Part model, mm, in its own coordinate system. A direction names the side the tool comes from. Give positions to 0.01 mm unless a question says otherwise; leave off trailing zeros. Loops run counter-clockwise (first coordinate to the right, second up) from the corner with the lowest first, then second, coordinate; pieces in that order, holes last. Notation, with made-up numbers: M 73,-28.75 L 122,-28.75 A12 cw 122,-11.75 Z; hole C -37.75,70.25 d3. An arc over 180 degrees is marked long. Answer in a Markdown table with one row per item.
from build123d import *

# Parameters (mm, degrees)
SKETCH1_R           = 2.5
BOSS_EXTRUDE1_DEPTH = 15
SKETCH3_W           = 4
SKETCH3_H           = 5
CUT_EXTRUDE1_START  = -1
CUT_EXTRUDE1_DEPTH  = 30
CHAMFER1_SIZE       = 0.5


with BuildPart() as part:
    # Sketch1 → Boss-Extrude1 (new body)
    with BuildSketch(Plane(origin=(0, 0, 0), x_dir=(1, 0, 0), z_dir=(0, 1, 0))):
        with Locations(Location((0, 0, 0), (0, 0, 270))):
            Circle(SKETCH1_R)
    extrude(amount=BOSS_EXTRUDE1_DEPTH)

    # Sketch3 → Revolve1 (revolve)
    with BuildSketch(Plane.XY, mode=Mode.PRIVATE) as revolve1_sk:
        with Locations((-2, -2.5)):
            Rectangle(SKETCH3_W, SKETCH3_H)
    revolve(revolve1_sk.sketch.rotate(Axis((0, -5, 0), (0, 1, 0)), 270), axis=Axis((0, -5, 0), (0, 1, 0)))

    # Sketch4 → Cut-Extrude1 (cut)
    with BuildSketch(Plane(origin=(0, 0, 0), x_dir=(1, 0, 0), z_dir=(0, 1, 0)).offset(CUT_EXTRUDE1_START)):
        Polygon((2.886751346, 0), (1.443375673, 2.5), (-1.443375673, 2.5), (-2.886751346, 0), (-1.443375673, -2.5), (1.443375673, -2.5), align=None)
    extrude(amount=-CUT_EXTRUDE1_DEPTH, mode=Mode.SUBTRACT)

    # Chamfer1
    chamfer1_edges = [part.edges().sort_by_distance(p)[0] for p in [
        (0, 0, 4),
        (0, -5, 4),
    ]]
    chamfer(chamfer1_edges, length=CHAMFER1_SIZE)


solid = part.part
(1) Saw through at A-A (y = -2). Write the cut outline in (x, z), plus the area to 3 significant figures.
Recorded:
| item | result |
|---|---|
| outline | C 0,0 d8; hole M -2.89,0 L -1.44,-2.5 L 1.44,-2.5 L 2.89,0 L 1.44,2.5 L -1.44,2.5 Z |
| area | 28.6 mm^2 |
(2) Saw through at B-B (x = 0). Write the cut outline in (y, z).
Recorded:
| item | result |
|---|---|
| outline | M -5,-3.5 L -4.5,-4 L -0.5,-4 L 0,-3.5 L 0,-2.5 L 15,-2.5 L 15,2.5 L 0,2.5 L 0,3.5 L -0.5,4 L -4.5,4 L -5,3.5 L -5,2.5 L -1,2.5 L -1,-2.5 L -5,-2.5 Z |
(3) Which spindle directions (+Z, -Z, +X, -X, +Y, -Y) get a long thin tool onto all of the face, cutting with end or side? Do faces 1 (the face through (-2.44, 7.4, -0.54)), 2 (the face through (-2.175, -2.972, 1.233)), 3 (the face through (0, 15, 0)). Say none if no direction does.
Recorded:
| item | result |
|---|---|
| face 1 | +Y |
| face 2 | -Y |
| face 3 | +Z, -Z, +X, -X, +Y |
(4) Pin check, flat tips, straight feed: pin 1 Ø3 at (y, z) = (12.5, 1.5) entering from +X; pin 2 Ø1.5 at (x, y) = (1.5, 9) entering from +Z. Stop position of each tip, or through.
Recorded:
| item | result |
|---|---|
| pin 1 | stops at x = 2.5 |
| pin 2 | stops at z = 2.38 |
(5) Drill centre lines: line 1 along Y through (x, z) = (3, 0.5); line 2 along X through (y, z) = (4, 0); line 3 along X through (y, z) = (-2.5, -0.75). Where is each one in solid material? Low to high.
Recorded:
| item | result |
|---|---|
| line 1 | y = -5 to 0 |
| line 2 | x = -2.5 to 2.5 |
| line 3 | x = -3.93 to -2.45, 2.45 to 3.93 |
(6) Saw through at C-C (y = 5.75). Write the cut outline in (x, z).
Recorded:
| item | result |
|---|---|
| outline | C 0,0 d5 |
(7) Pull direction X, two halves, no side cores. Call faces 4 (the face through (2.155, -2.972, 1.267)), 5 (the face through (-2, -5, 2)), 6 (the face through (3.905, -2.472, 0.867)): +X half, -X half, draft (parallel to the pull), parting line (faces both ways), or undercut.
Recorded:
| item | result |
|---|---|
| face 4 | undercut |
| face 5 | draft |
| face 6 | parting line |
